Part print with two shaded views. Sizes in mm from the minimum x, y, z corner. A direction names the side the tool comes from. Coordinates: 2 decimals unless noted, no trailing zeros. Order: outer loops, then holes, each group sorted by start corner. A loop starts at its lowest first (then second) coordinate and runs counter-clockwise, first axis right, second up. Notation, with made-up numbers: (73.5, 6) - (90.5, 6) arc R17 cw to (90.5, 29) - close; hole circle Ø4 at (28, 79). An arc over 180 degrees is marked (long way). One line per item, written item: value.
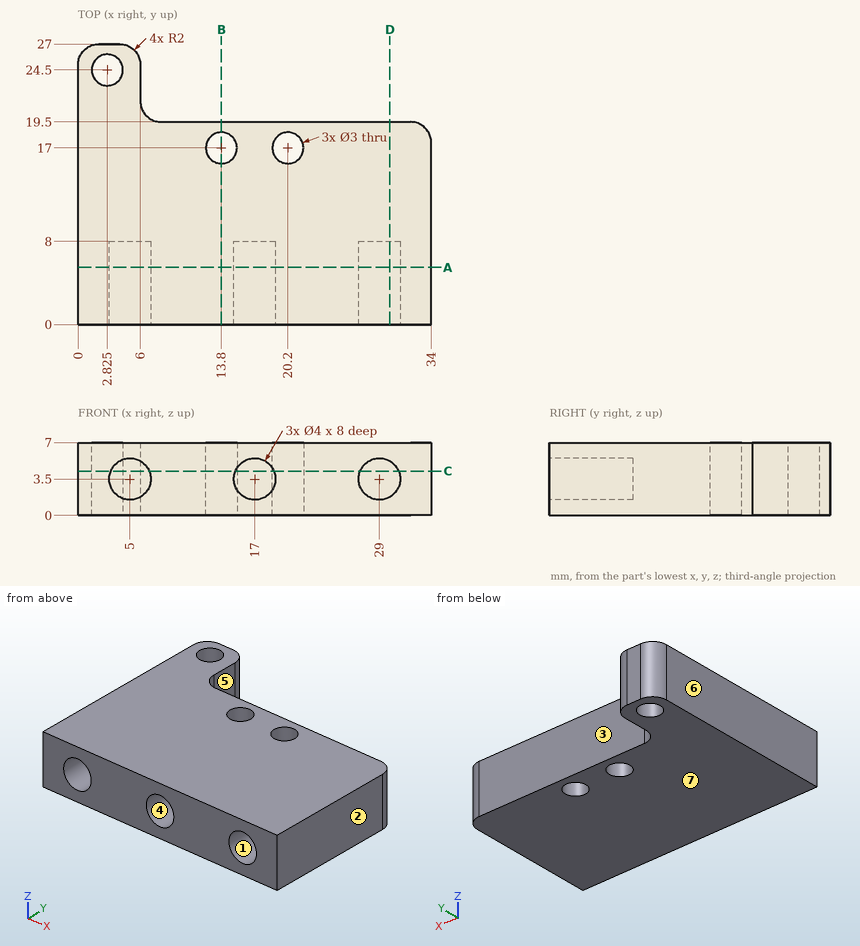
1. 3-axis set-ups, long thin cutter, end or side, ignore diameter. For the marked faces 1, 2 and 3: which of +Z, -Z, +X, -X, +Y, -Y reach the whole face in a straight line?
Values found:
face 1: -Y
face 2: +Z, -Z, +X, +Y, -Y
face 3: +Z, -Z, +X, +Y
2. Band-saw the part on B-B, the plane x = 13.8. Give the cut face in (y, z), and give its area (4 significant figures).
Values found:
outline: (0, 0) - (15.5, 0) - (15.5, 7) - (0, 7) - close; (18.5, 0) - (19.5, 0) - (19.5, 7) - (18.5, 7) - close
area: 115.5 mm2
3. Probe line 1 along Z through (x, y) = (17, 4.5); line 2 along Y through (x, z) = (10, 1); line 3 along Y through (x, z) = (18, 3.5). List the from-to ranges inside material, lowest first.
Values found:
line 1: z = 0 to 1.5, 5.5 to 7
line 2: y = 0 to 19.5
line 3: y = 8 to 19.5
4. Flat gauge pins, fed straight in: P1, Ø3, axis at x = 29, z = 3.5, coming from the +Y side; P2, Ø2, axis at x = 29.5, z = 3.5, coming from the -Y side; P3, Ø1.8, axis at y = 23, z = 5, coming from the +X side. Where does each tip first touch, or does it go through?
Values found:
P1: stops at y = 19.5
P2: stops at y = 8
P3: stops at x = 6
5. Band-saw the part on A-A, the plane y = 5.5. Give the cut face in (x, z), and give its area (3 significant figures).
Values found:
outline: (0, 0) - (34, 0) - (34, 7) - (0, 7) - close; hole circle Ø4 at (5, 3.5); hole circle Ø4 at (17, 3.5); hole circle Ø4 at (29, 3.5)
area: 200 mm2
6. Band-saw the part on C-C, the plane z = 4.25. Give the cut face in (x, y) (3 decimals), and give its area (3 significant figures).
Values found:
outline: (0, 0) - (3.146, 0) - (3.146, 8) - (6.854, 8) - (6.854, 0) - (15.146, 0) - (15.146, 8) - (18.854, 8) - (18.854, 0) - (27.146, 0) - (27.146, 8) - (30.854, 8) - (30.854, 0) - (34, 0) - (34, 17.5) arc R2 ccw to (32, 19.5) - (8, 19.5) arc R2 cw to (6, 21.5) - (6, 25) arc R2 ccw to (4, 27) - (2, 27) arc R2 ccw to (0, 25) - close; hole circle Ø3 at (2.825, 24.5); hole circle Ø3 at (13.8, 17); hole circle Ø3 at (20.2, 17)
area: 596 mm2
7. Band-saw the part on D-D, the plane x = 30. Give the cut face in (y, z).
Values found:
outline: (0, 0) - (19.5, 0) - (19.5, 7) - (0, 7) - (0, 5.23) - (8, 5.23) - (8, 1.77) - (0, 1.77) - close
8. Two-plate mould, pull along X, no slides. Class the marked faces 4, 5, 6 and 7: pulls with the +X half, pulls with the -X half, needs draft (parallel to the pull), parting line crosses it, or undercut.
Values found:
face 4: undercut
face 5: pulls with the +X half
face 6: pulls with the -X half
face 7: needs draft
